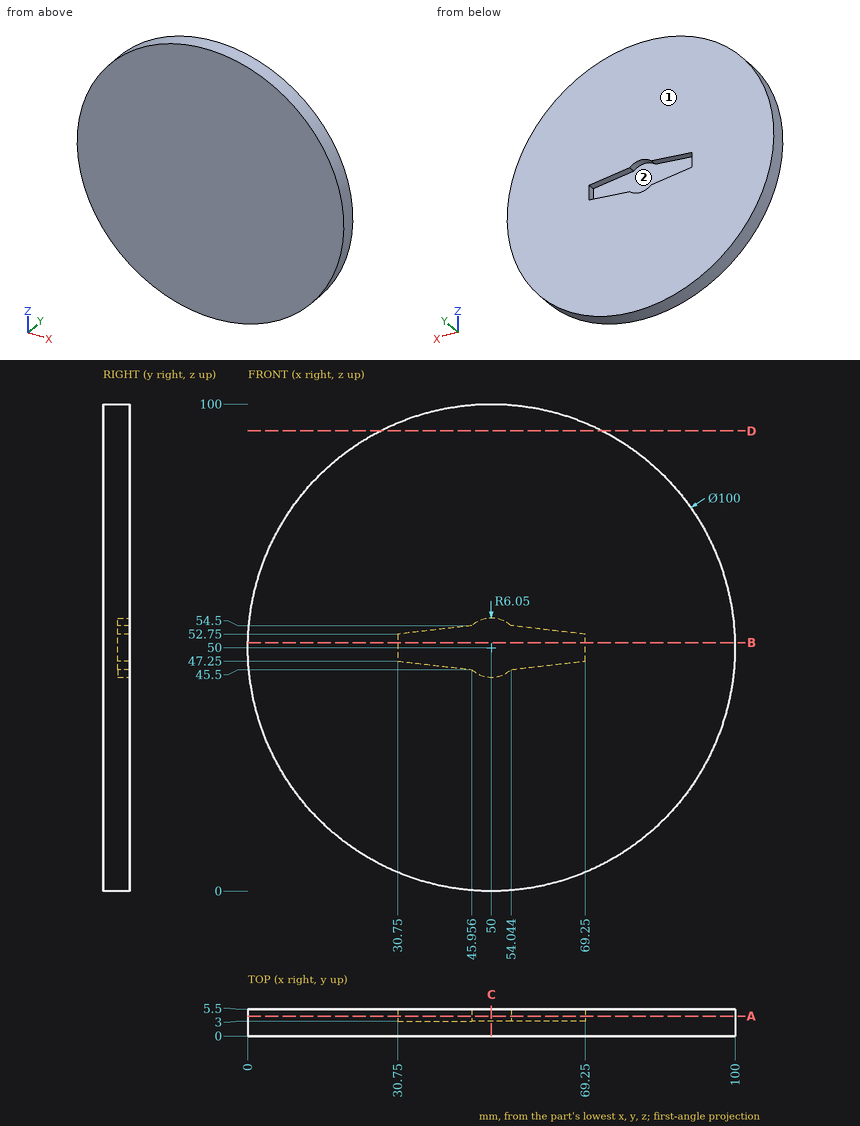
Print and shaded views of the part. All mm, measured from the part's lowest x, y and z. A direction names the side the tool comes from. Coordinates: 2 decimals unless noted, no trailing zeros. Loops run counter-clockwise (first coordinate to the right, second up) from the corner with the lowest first, then second, coordinate; pieces in that order, holes last. Notation, with made-up numbers: M 37,55.5 L 79,55.5 A20 ccw 79,61.5 Z; hole C -32.5,-21 d1. An arc over 180 degrees is marked long. Use a Markdown table: item, result. Add a question column.
Q1. Probe L1, parallel to Y at x = 31, z = 49.5; L2, parallel to Z at x = 38, y = 4.65; L3, parallel to Z at x = 40, y = 4.9 (1 decimal). List the from-to ranges inside material, lowest first.
Q2. Cut at C-C (x = 50). Write the cut outline in (y, z), and give its area (3 significant figures).
Q3. Which spindle directions (+Z, -Z, +X, -X, +Y, -Y) get a long thin tool onto all of the face, cutting with end or side? Do the marked faces 1 and 2. Say none if no direction does.
Q4. Cut at B-B (z = 51). Write the cut outline in (x, y), and give its area (3 significant figures).
Q5. Pin check, flat tips, straight feed: P1, Ø2, axis at x = 44, y = 3, coming from the +Z side; P2, Ø1, axis at y = 4.5, z = 88, coming from the -X side; P3, Ø3.5, axis at x = 50, z = 47.5, coming from the +Y side. Stop position of each tip, or through.
Q6. Cut at A-A (y = 4.1). Write the cut outline in (x, z).
Q7. Cut at D-D (z = 94.5). Write the cut outline in (x, y).
Worked out:
| question | item | result |
|---|---|---|
| 1 | L1 | y = 0 to 3 |
| 1 | L2 | z = 1.46 to 46.42, 53.58 to 98.54 |
| 1 | L3 | z = 1 to 46.2, 53.8 to 99 |
| 2 | outline | M 0,0 L 5.5,0 L 5.5,43.95 L 3,43.95 L 3,56.05 L 5.5,56.05 L 5.5,100 L 0,100 Z |
| 2 | area | 520 mm2 |
| 3 | face 1 | +Z, -Z, +X, -X, +Y |
| 3 | face 2 | +Y |
| 4 | outline | M 0.01,0 L 99.99,0 L 99.99,5.5 L 69.25,5.5 L 69.25,3 L 30.75,3 L 30.75,5.5 L 0.01,5.5 Z |
| 4 | area | 454 mm2 |
| 5 | P1 | stops at z = 99.75 |
| 5 | P2 | stops at x = 16.93 |
| 5 | P3 | stops at y = 3 |
| 6 | outline | C 50,50 d100; hole M 30.75,47.25 L 45.96,45.5 A6.05 ccw 54.04,45.5 L 69.25,47.25 L 69.25,52.75 L 54.04,54.5 A6.05 ccw 45.96,54.5 L 30.75,52.75 Z |
| 7 | outline | M 27.2,0 L 72.8,0 L 72.8,5.5 L 27.2,5.5 Z |
